```python
from build123d import *

# Parameters (mm, degrees)
SKETCH3_W           = 20
SKETCH3_H           = 40
BOSS_EXTRUDE1_DEPTH = 3
SKETCH4_R           = 6.35
SKETCH4_R_2         = 3.175
CUT_EXTRUDE1_DEPTH  = 5
FILLET2_RADIUS      = 10
FILLET2_LENGTH      = 3
FILLET3_RADIUS      = 10
FILLET3_LENGTH      = 3


with BuildPart() as part:
    # Sketch3 → Boss-Extrude1 (new body)
    with BuildSketch(Plane(origin=(0, 0, 0), x_dir=(0, 0, -1), z_dir=(1, 0, 0))):
        Rectangle(SKETCH3_W, SKETCH3_H)
    extrude(amount=BOSS_EXTRUDE1_DEPTH)

    # Sketch4 → Cut-Extrude1 (cut)
    with BuildSketch(Plane(origin=(3, 0, 0), x_dir=(0, 0, -1), z_dir=(1, 0, 0))):
        with Locations((0, 10)):
            Circle(SKETCH4_R)
        with Locations((0, -10)):
            Circle(SKETCH4_R_2)
    extrude(amount=-CUT_EXTRUDE1_DEPTH, mode=Mode.SUBTRACT)

    # Fillet2: full round fillet: the end face becomes a half cylinder, R = half its width
    fillet2_face = Plane((1.5, -20, 0), x_dir=(-1, 0, 0), z_dir=(0, -1, 0))  # on the end face: x along it, z out of the body
    fillet2_slab = fillet2_face.offset(-FILLET2_RADIUS / 2) * Box(FILLET2_LENGTH, 2 * FILLET2_RADIUS, FILLET2_RADIUS, mode=Mode.PRIVATE)  # the body's end, R deep
    fillet2_round = Plane((1.5, -10, 0), x_dir=(0, -1, 0), z_dir=(-1, 0, 0)) * Cylinder(FILLET2_RADIUS, FILLET2_LENGTH, mode=Mode.PRIVATE)  # its axis R under the face
    add(fillet2_slab - fillet2_round, mode=Mode.SUBTRACT)

    # Fillet3: full round fillet: the end face becomes a half cylinder, R = half its width
    fillet3_face = Plane((1.5, 20, 0), x_dir=(-1, 0, 0), z_dir=(0, 1, 0))  # on the end face: x along it, z out of the body
    fillet3_slab = fillet3_face.offset(-FILLET3_RADIUS / 2) * Box(FILLET3_LENGTH, 2 * FILLET3_RADIUS, FILLET3_RADIUS, mode=Mode.PRIVATE)  # the body's end, R deep
    fillet3_round = Plane((1.5, 10, 0), x_dir=(0, 1, 0), z_dir=(-1, 0, 0)) * Cylinder(FILLET3_RADIUS, FILLET3_LENGTH, mode=Mode.PRIVATE)  # its axis R under the face
    add(fillet3_slab - fillet3_round, mode=Mode.SUBTRACT)


solid = part.part
```
Read the model definition and answer for the solid it produces. Units are mm, in the model's axes. Coordinates: 2 decimals unless noted, no trailing zeros. Write each loop counter-clockwise with the first axis right and the second up, starting at its lowest first coordinate (ties: lowest second). Pieces come first, ordered by that corner, then holes. Notation, with made-up numbers: (5, 58.25) - (13, 58.25) arc R19 cw to (13, 68.25) - close; hole circle Ø5 at (9.25, 47). An arc over 180 degrees is marked (long way). Answer as a JSON object with one key per item and string values. Group by question number.
1. A cutting plane is placed at C-C (x = 1.9). Determine the outline of the cut face in (y, z) (3 decimals), plus the area to 3 significant figures.
2. A cutting plane is placed at B-B (y = -10.5). Determine the outline of the cut face in (x, z).
3. A cutting plane is placed at D-D (z = 4.5). Determine the outline of the cut face in (x, y).
4. This flat-tipped pin is pushed along its axis until it touches: P1, Ø11.5, axis at y = 10, z = 0, coming from the +X side. Where does it stop, or does it pass through?
5. The mould has two halves that part along Z. Classify faces 1 (the flat face through (3, 0, 0)), 2 (the cylindrical face through (1.52, 3.8, 1.38)), 3 (the cylindrical face through (1, 20, 0)), 4 (the flat face through (1, 0, -10)): +Z half, -Z half, draft (parallel to the pull), parting line (faces both ways), or undercut.
6. Consider L1, parallel to Y at x = 2.1, z = 0 (3 decimals); L2, parallel to Y at x = 1.3, z = -2.5; L3, parallel to Y at x = 1.65, z = 4.25. Determine where each line is inside the solid, lowest interval first. Write a range as [from, to].
7. A cutting plane is placed at A-A (z = 0). Determine the outline of the cut face in (x, y) (3 decimals).
Worked out:
{
 "1": {"outline": "(-10, -10) - (10, -10) arc R10 ccw to (10, 10) - (-10, 10) arc R10 ccw to start; hole circle Ø6.35 at (-10, 0); hole circle Ø12.7 at (10, 0)", "area": "556 mm²"},
 "2": {"outline": "(0, -9.99) - (3, -9.99) - (3, -3.14) - (0, -3.14) - close; (0, 3.14) - (3, 3.14) - (3, 9.99) - (0, 9.99) - close"},
 "3": {"outline": "(0, -18.93) - (3, -18.93) - (3, 5.52) - (0, 5.52) - close; (0, 14.48) - (3, 14.48) - (3, 18.93) - (0, 18.93) - close"},
 "4": {"P1": "passes through"},
 "5": {"face 1": "draft", "face 2": "undercut", "face 3": "parting line", "face 4": "-Z half"},
 "6": {"L1": "y = [-20, -13.175], [-6.825, 3.65], [16.35, 20]", "L2": "y = [-19.68, -11.96], [-8.04, 4.16], [15.84, 19.68]", "L3": "y = [-19.05, 5.28], [14.72, 19.05]"},
 "7": {"outline": "(0, -20) - (3, -20) - (3, -13.175) - (0, -13.175) - close; (0, -6.825) - (3, -6.825) - (3, 3.65) - (0, 3.65) - close; (0, 16.35) - (3, 16.35) - (3, 20) - (0, 20) - close"}
}
